Source: CAD feature listing. Evaluate the final solid. Frame: model axes, mm. A direction names the side the tool comes from. Coordinates: 2 decimals unless noted, no trailing zeros. Write each loop counter-clockwise with the first axis right and the second up, starting at its lowest first coordinate (ties: lowest second). Pieces come first, ordered by that corner, then holes. Notation, with made-up numbers: M 9.5,8 L 27.5,8 A18 ccw 27.5,25 Z; hole C 46,-12 d11. An arc over 180 degrees is marked long. Answer as CSV lines item,"result". Start each with the question number.
1. Reachability of faces 5 (the face through (33, -1.5, 19)), 6 (the face through (33, 0, 18)) from +Z, -Z, +X, -X, +Y, -Y: full face, straight path, thin tool, end or side. Return the list, or none.
2. Section A-A on z = 20. Return the cut outline in (x, y).
3. Section C-C on y = -29. Return the cut outline in (x, z).
4. Mould query, pull axis Z, two halves, no side actions, for faces 1 (the face through (33.44, -35.6, 34.14)), 2 (the face through (33, -19, 0)), 3 (the face through (0, -19, 18)), 4 (the face through (33, -36.5, 17)). Classes: pulls with the +Z half, pulls with the -Z half, needs draft (parallel to the pull), parting line crosses it, or undercut.
5. Line query: probe 1 along X at (y, z) = (-2, 31); probe 2 along Y at (x, z) = (29.5, 32); probe 3 along Z at (x, y) = (53, -26.5). Output: solid intervals per line, ascending. Write a range as [from, to].
6. Section D-D on z = 33. Return the cut outline in (x, y).
7. Contact query for flat-ended pins moving along their axis: pin 1 Ø10 at (x, y) = (20, -12) entering from -Z; pin 2 Ø2 at (x, y) = (23, -16) entering from +Z. Output: stop coordinate, or through.
```python
from build123d import *

# Parameters (mm, degrees)
SKETCH_1_W      = 66
SKETCH_1_H      = 38
EXTRUDE_1_DEPTH = 1.5
SKETCH_2_W      = 66
SKETCH_2_H      = 38
SKETCH_2_W_2    = 63
SKETCH_2_H_2    = 35
EXTRUDE_2_DEPTH = 35
SKETCH_3_W      = 63
SKETCH_3_H      = 1.5
EXTRUDE_3_DEPTH = 3
FILLET_1_R      = 3


with BuildPart() as part:
    # 草图1 → 凸台-拉伸1 (new body)
    with BuildSketch(Plane.XY):
        with Locations((33, -19)):
            Rectangle(SKETCH_1_W, SKETCH_1_H)
    extrude(amount=EXTRUDE_1_DEPTH)

    # 草图2 → 凸台-拉伸2 (add)
    with BuildSketch(Plane.XY.offset(1.5)):
        with Locations((33, -19)):
            Rectangle(SKETCH_2_W, SKETCH_2_H)
        with Locations((33, -19)):
            Rectangle(SKETCH_2_W_2, SKETCH_2_H_2, mode=Mode.SUBTRACT)
    extrude(amount=EXTRUDE_2_DEPTH)

    # 草图3 → 凸台-拉伸3 (add)
    with BuildSketch(Plane(origin=(0, -36.5, 0), x_dir=(1, 0, 0), z_dir=(0, 1, 0))):
        with Locations((33, -35.75)):
            Rectangle(SKETCH_3_W, SKETCH_3_H)
    extrude(amount=EXTRUDE_3_DEPTH)

    # 圆角1
    fillet_1_edges = [part.edges().sort_by_distance(p)[0] for p in [
        (33, -36.5, 35),
    ]]
    fillet(fillet_1_edges, radius=FILLET_1_R - 0.0001)  # a hair under: the kernel refuses the full size


solid = part.part
```
Values:
1,face 5,"+Z"
1,face 6,"+Z, -Z, +X, -X, +Y"
2,outline,"M 0,-38 L 66,-38 L 66,0 L 0,0 Z; hole M 1.5,-36.5 L 64.5,-36.5 L 64.5,-1.5 L 1.5,-1.5 Z"
3,outline,"M 0,0 L 66,0 L 66,36.5 L 64.5,36.5 L 64.5,1.5 L 1.5,1.5 L 1.5,36.5 L 0,36.5 Z"
4,face 1,"undercut"
4,face 2,"pulls with the -Z half"
4,face 3,"needs draft"
4,face 4,"undercut"
5,probe 1,"[0, 1.5], [64.5, 66]"
5,probe 2,"[-38, -36.5], [-1.5, 0]"
5,probe 3,"[0, 1.5]"
6,outline,"M 0,-38 L 66,-38 L 66,0 L 0,0 Z; hole M 1.5,-36.33 L 64.5,-36.33 L 64.5,-1.5 L 1.5,-1.5 Z"
7,pin 1,"z = 0"
7,pin 2,"z = 1.5"
